The figure shows three views and two pictorial views of one solid part (mm, origin at its lowest corner). Answer the questions. Give positions to 0.01 mm unless a question says otherwise; leave off trailing zeros. Loops run counter-clockwise (first coordinate to the right, second up) from the corner with the lowest first, then second, coordinate; pieces in that order, holes last. Notation, with made-up numbers: M -33.5,71 L 11.5,71 A25 ccw 11.5,101 Z; hole C -30,-33 d6. An arc over 180 degrees is marked long. Answer in a Markdown table with one row per item. Add a question column.
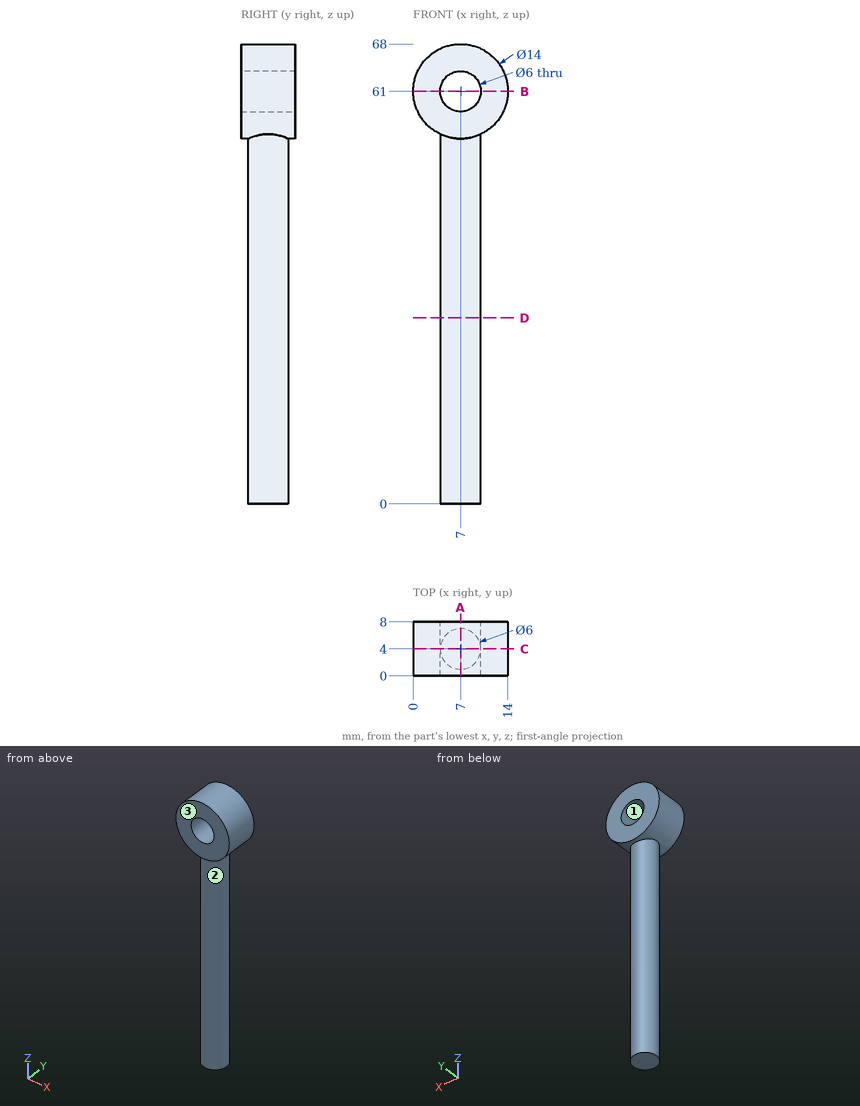
(1) Section B-B, the plane z = 61 is taken. Determine the outline of the cut face in (x, y).
(2) Consider line 1 along X through (y, z) = (4.75, 61); line 2 along Z through (x, y) = (8.25, 1.75); line 3 along Z through (x, y) = (4.75, 1.5). Determine where each line is inside the solid, lowest interval first. Write a range as from..to.
(3) Section A-A, the plane x = 7 is taken. Determine the outline of the cut face in (y, z).
(4) Section D-D, the plane z = 27.5 is taken. Determine the outline of the cut face in (x, y).
(5) Each of these flat-tipped pins is pushed along its axis until it touches: P1, Ø1, axis at x = 11.5, y = 4.5, coming from the +Z side; P2, Ø3, axis at x = 12, y = 6, coming from the +Z side; P3, Ø6, axis at x = 2.5, z = 39.5, coming from the -Y side. Where does it stop, or does it pass through?
(6) The mould has two halves that part along X. Classify the marked faces 1, 2 and 3: pulls with the +X half, pulls with the -X half, needs draft (parallel to the pull), parting line crosses it, or undercut.
(7) Section C-C, the plane y = 4 is taken. Determine the outline of the cut face in (x, z), and give its area (3 significant figures).
Numbers:
| question | item | result |
|---|---|---|
| 1 | outline | M 0,0 L 4,0 L 4,8 L 0,8 Z; M 10,0 L 14,0 L 14,8 L 10,8 Z |
| 2 | line 1 | x = 0..4, 10..14 |
| 2 | line 2 | z = 0..58.27, 63.73..67.89 |
| 2 | line 3 | z = 54.37..59.02, 62.98..67.63 |
| 3 | outline | M 0,54 L 1,54 L 1,0 L 7,0 L 7,54 L 8,54 L 8,58 L 0,58 Z; M 0,64 L 8,64 L 8,68 L 0,68 Z |
| 4 | outline | C 7,4 d6 |
| 5 | P1 | stops at z = 66.74 |
| 5 | P2 | stops at z = 67.06 |
| 5 | P3 | stops at y = 1.4 |
| 6 | face 1 | undercut |
| 6 | face 2 | parting line crosses it |
| 6 | face 3 | needs draft |
| 7 | outline | M 4,0 L 10,0 L 10,54.68 A7 ccw long 4,54.68 Z; hole C 7,61 d6 |
| 7 | area | 451 mm² |
